from build123d import *

# Parameters (mm, degrees)
SKETCH1_R           = 2.5
BOSS_EXTRUDE1_DEPTH = 5
SKETCH2_W           = 25
SKETCH2_H           = 10
BOSS_EXTRUDE2_DEPTH = 15
SKETCH3_W           = 6
SKETCH3_H           = 15
CUT_EXTRUDE1_DEPTH  = 15
FILLET1_R           = 10
FILLET2_R           = 10
FILLET3_R           = 5
SKETCH4_W           = 10
SKETCH4_H           = 10
BOSS_EXTRUDE3_DEPTH = 10
FILLET4_R           = 5
SKETCH5_R           = 2.5
CUT_EXTRUDE2_DEPTH  = 10


# Some blends are built 0.0001 mm under size
with BuildPart() as part:
    # Sketch1 → Boss-Extrude1 (new, symmetric)
    with BuildSketch(Plane.XY):
        with BuildLine():
            ThreePointArc((-7.5, 0), (0, -7.5), (7.5, 0))
            Line((7.5, 0), (7.5, 25))
            ThreePointArc((7.5, 25), (0, 32.5), (-7.5, 25))
            Line((-7.5, 25), (-7.5, 0))
        make_face()
        Circle(SKETCH1_R, mode=Mode.SUBTRACT)
        with Locations((0, 25)):
            Circle(SKETCH1_R, mode=Mode.SUBTRACT)
    extrude(amount=BOSS_EXTRUDE1_DEPTH, both=True)

    # Sketch2 → Boss-Extrude2 (add)
    with BuildSketch(Plane.ZY.offset(7.5)):
        with Locations((0, 12.5)):
            Rectangle(SKETCH2_W, SKETCH2_H)
    extrude(amount=BOSS_EXTRUDE2_DEPTH)

    # Sketch3 → Cut-Extrude1 (cut)
    with BuildSketch(Plane(origin=(0, 17.5, 0), x_dir=(1, 0, 0), z_dir=(0, 1, 0))):
        with Locations((-15, 0)):
            Rectangle(SKETCH3_W, SKETCH3_H)
    extrude(amount=-CUT_EXTRUDE1_DEPTH, mode=Mode.SUBTRACT)

    # Fillet1
    # the kernel refuses this fillet: 10 mm, written as the material it adds along each edge
    with BuildSketch(Plane(origin=(-7.5, 17.5, -5), x_dir=(1, 0, 0), z_dir=(0, -1, 0))) as fillet1_piece_1:
        with BuildLine():
            CenterArc((9.682458366, -10), FILLET1_R, 90, 75.522487814)
            Line((0, -7.5), (0, 0))
            Line((0, 0), (9.682458366, 0))
        make_face()
    extrude(amount=10)
    with BuildSketch(Plane(origin=(-7.5, 17.5, 5), x_dir=(1, 0, 0), z_dir=(0, -1, 0))) as fillet1_piece_2:
        with BuildLine():
            CenterArc((9.682458366, 10), FILLET1_R, 194.477512186, 75.522487814)
            Line((0, 7.5), (0, 0))
            Line((0, 0), (9.682458366, 0))
        make_face()
    extrude(amount=10)
    # the kernel refuses this fillet: 10 mm, written as the material it takes off along each edge
    with BuildSketch(Plane(origin=(-22.5, -17.5, 12.5), x_dir=(1, 0, 0), z_dir=(0, 1, 0)), Plane(origin=(-22.5, 42.5, -12.5), x_dir=(1, 0, 0), z_dir=(0, -1, 0))) as fillet1_2_piece_1:
        with BuildLine():
            CenterArc((FILLET1_R, FILLET1_R), FILLET1_R, 180, 90)
            Line((0, FILLET1_R), (0, 0))
            Line((0, 0), (FILLET1_R, 0))
        make_face()
    extrude(amount=60, mode=Mode.SUBTRACT)

    # Fillet2
    # the kernel refuses this fillet: 10 mm, written as the material it takes off along each edge
    with BuildSketch(Plane(origin=(-7.5, 30, -12.5), x_dir=(-1.0, 0, 1.525535253676709e-12), z_dir=(0, -1, 0))) as fillet2_piece_1:
        with BuildLine():
            CenterArc((5.967480043, -9.953089087), FILLET2_R, 95.55193659, 45.937826444)
            Line((-1.857489161, -3.726544543), (-2.013988545, -3.602013652))
            ThreePointArc((-2.013988545, -3.602013652), (-0.911634188, -1.871800915), (-0.193649167, 0.05))
            Line((-0.193649167, 0.05), (0, 0.2))
            ThreePointArc((0, 0.2), (2.5, 0.2), (4.980650399, 0.199061782))
            Line((4.980650399, 0.199061782), (5, 0))
        make_face()
    extrude(amount=35, mode=Mode.SUBTRACT)
    with BuildSketch(Plane(origin=(-7.5, -5, 12.5), x_dir=(0.4461021341851978, 0, -0.8949820589684531), z_dir=(0, 1, 0))) as fillet2_piece_2:
        with BuildLine():
            CenterArc((6.245730581, 9.780881859), FILLET2_R, 212.045811166, 45.937826444)
            Line((-2.230510671, 4.474910295), (-2.400035496, 4.368790864))
            ThreePointArc((-2.400035496, 4.368790864), (-1.294251747, 2.148234721), (-0.178996412, -0.089220427))
            Line((-0.178996412, -0.089220427), (0.041638204, -0.195617637))
            ThreePointArc((0.041638204, -0.195617637), (2.081910194, 0.019118141), (4.122182183, -0.195617637))
            Line((4.122182183, -0.195617637), (4.163820387, 0))
        make_face()
    extrude(amount=35, mode=Mode.SUBTRACT)

    # Fillet3
    fillet3_edges = [part.edges().sort_by_distance(p)[0] for p in [
        (-18, 12.5, 7.5),
        (-18, 12.5, -7.5),
    ]]
    fillet(fillet3_edges, radius=FILLET3_R)

    # Sketch4 → Boss-Extrude3 (add)
    with BuildSketch(Plane(origin=(7.5, 0, 0), x_dir=(0, 0, -1), z_dir=(1, 0, 0))):
        with Locations((0, 12.5)):
            Rectangle(SKETCH4_W, SKETCH4_H)
    extrude(amount=BOSS_EXTRUDE3_DEPTH)

    # Fillet4
    fillet4_edges = [part.edges().sort_by_distance(p)[0] for p in [
        (17.5, 12.5, -5),
        (17.5, 12.5, 5),
    ]]
    fillet(fillet4_edges, radius=FILLET4_R - 0.0001)  # a hair under: the kernel refuses the full size

    # Sketch5 → Cut-Extrude2 (cut)
    with BuildSketch(Plane(origin=(0, 17.5, 0), x_dir=(1, 0, 0), z_dir=(0, 1, 0))):
        with Locations(Location((12.5, 0, 0), (0, 0, 270))):
            Circle(SKETCH5_R)
    extrude(amount=-CUT_EXTRUDE2_DEPTH, mode=Mode.SUBTRACT)


solid = part.part
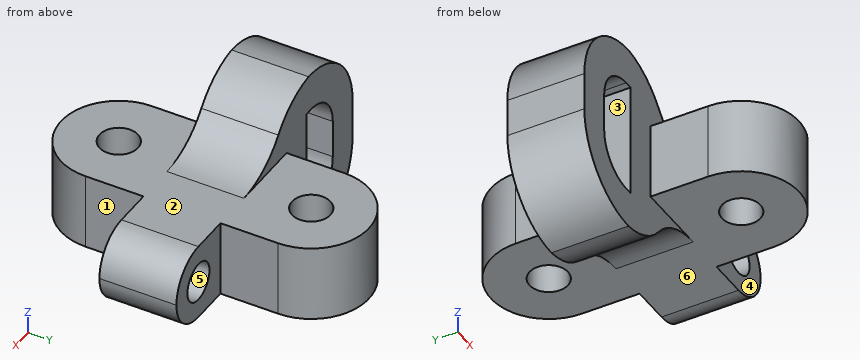
Design review of the part built by this model. Coordinates are the model's own, in mm. Face numbers are marked on the shaded views. A direction names the side the tool comes from. Round coordinates to 2 decimals unless told otherwise and drop trailing zeros. Write each loop counter-clockwise with the first axis right and the second up, starting at its lowest first coordinate (ties: lowest second). Pieces come first, ordered by that corner, then holes.
Item 1: Consider section C-C on z = 4. Give the boundary of the cut face in (x, y).
Item 2: For the marked faces 1, 2 and 3, list the 3-axis set-ups (+Z, -Z, +X, -X, +Y, -Y) from which the entire face can be reached by the end or side of a thin tool; tool diameter is ignored.
Item 3: Draft analysis for pull direction Z (two halves, no side actions). For the marked faces 4, 5 and 6, state which applies: released by +Z, released by -Z, zero draft, split by the parting line, or undercut.
Item 4: Consider section B-B on y = 15. Count the separate pieces of the cut face and the enclosed holes in it, and give its area (3 significant figures).
Item 5: Consider section D-D on x = -14. Give the boundary of the cut face in (y, z), and give its area (3 significant figures).
Item 6: Consider section A-A on x = 0. Give the boundary of the cut face in (y, z).
Item 7: For pin 1 Ø5 at (y, z) = (7, 9) entering from +X; pin 2 Ø3 at (x, y) = (-2.5, 15.5) entering from +Z; pin 3 Ø2 at (y, z) = (22.5, -1) entering from -X; pin 4 Ø3 at (x, y) = (0, 0) entering from +Z, all flat-tipped, find the tip position at first contact; note any pin that passes through.
Item 8: Wall thickness on L1, parallel to X at y = 13.5, z = 0; L2, parallel to Y at x = 0, z = 0.5; L3, parallel to Y at x = -1, z = 3: over which ranges is each line inside the solid? List them lowest first.
Check values:
1. outline: (-22.39, 7.5) - (-17.77, 7.5) - (-17.77, 17.5) - (-22.39, 17.5) - close; (-12, 7.5) - (-7.5, 7.5) - (-7.5, 0) arc R7.5 ccw to (7.5, 0) - (7.5, 7.5) - (15.5, 7.5) - (15.5, 17.5) - (7.5, 17.5) - (7.5, 25) arc R7.5 ccw to (-7.5, 25) - (-7.5, 17.5) - (-12, 17.5) - close; hole circle Ø5 at (0, 0); hole circle Ø5 at (0, 25)
2. face 1: +Z, -Z, +X, -Y
2. face 2: +Z, +X
2. face 3: +Y, -Y
3. face 4: zero draft
3. face 5: undercut
3. face 6: released by -Z
4. separate pieces: 1
4. enclosed holes: 2
4. area: 501 mm2
5. outline: (7.5, -12.39) - (17.5, -12.39) - (17.5, -7.4) - (7.5, -7.4) - close; (7.5, 7.4) - (17.5, 7.4) - (17.5, 12.39) - (7.5, 12.39) - close
5. area: 99.8 mm2
6. outline: (-7.5, -5) - (-2.5, -5) - (-2.5, 5) - (-7.5, 5) - close; (2.5, -5) - (7.5, -5) - (7.5, -5.24) - (17.5, -5.24) - (17.5, -5) - (22.5, -5) - (22.5, 5) - (17.5, 5) - (17.5, 5.24) - (7.5, 5.24) - (7.5, 5) - (2.5, 5) - close; (27.5, -5) - (32.5, -5) - (32.5, 5) - (27.5, 5) - close
7. pin 1: stops at x = -3.17
7. pin 2: stops at z = 7.14
7. pin 3: stops at x = -7.5
7. pin 4: passes through
8. L1: x = -22.5 to -18, -12 to 10, 15 to 17.5
8. L2: y = -7.5 to -2.5, 2.5 to 22.5, 27.5 to 32.5
8. L3: y = -7.43 to -2.29, 2.29 to 22.71, 27.29 to 32.43
